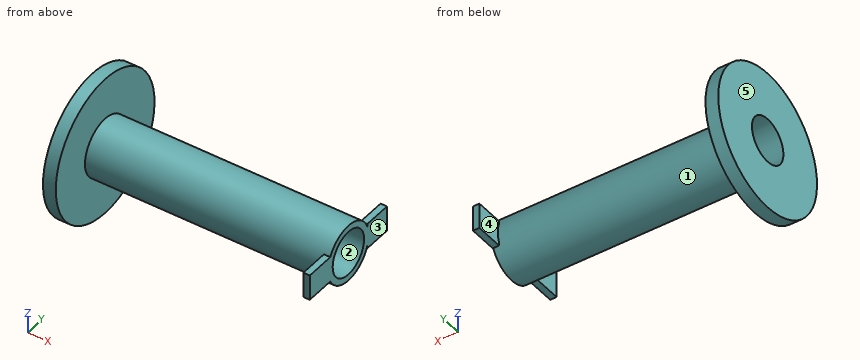
```python
from build123d import *

# Parameters (mm, degrees)
SKETCH2_R               = 55
BOSS_EXTRUDE1_DEPTH     = 10
SKETCH3_R               = 22.5
BOSS_EXTRUDE2_DEPTH     = 190
SKETCH4_R               = 17.5
CUT_EXTRUDE1_DEPTH      = 1
CUT_EXTRUDE1_DEPTH_BACK = 201
SKETCH9_W               = 20
SKETCH9_H               = 22
BOSS_EXTRUDE3_DEPTH     = 5
SKETCH10_W              = 20
SKETCH10_H              = 23
BOSS_EXTRUDE4_DEPTH     = 5


with BuildPart() as part:
    # Sketch2 → Boss-Extrude1 (new body)
    with BuildSketch(Plane(origin=(0, 0, 0), x_dir=(0, 0, -1), z_dir=(1, 0, 0))):
        Circle(SKETCH2_R)
    extrude(amount=BOSS_EXTRUDE1_DEPTH)

    # Sketch3 → Boss-Extrude2 (add)
    with BuildSketch(Plane(origin=(10, 0, 0), x_dir=(0, 0, -1), z_dir=(1, 0, 0))):
        Circle(SKETCH3_R)
    extrude(amount=BOSS_EXTRUDE2_DEPTH)

    # Sketch4 → Cut-Extrude1 (cut, two sides)
    with BuildSketch(Plane.ZY) as cut_extrude1_sk:
        Circle(SKETCH4_R)
    extrude(amount=CUT_EXTRUDE1_DEPTH, mode=Mode.SUBTRACT)
    extrude(cut_extrude1_sk.sketch, amount=-CUT_EXTRUDE1_DEPTH_BACK, mode=Mode.SUBTRACT)

    # Sketch9 → Boss-Extrude3 (add)
    with BuildSketch(Plane(origin=(200, 0, 0), x_dir=(0, 0, -1), z_dir=(1, 0, 0))):
        with Locations((0, 32)):
            Rectangle(SKETCH9_W, SKETCH9_H)
    extrude(amount=-BOSS_EXTRUDE3_DEPTH)

    # Sketch10 → Boss-Extrude4 (add)
    with BuildSketch(Plane(origin=(200, 0, 0), x_dir=(0, 0, -1), z_dir=(1, 0, 0))):
        with Locations((0, -31.5)):
            Rectangle(SKETCH10_W, SKETCH10_H)
    extrude(amount=-BOSS_EXTRUDE4_DEPTH)


solid = part.part
```
The model under review builds one solid part; all positions refer to its coordinate system, in mm. Face numbers are marked on the shaded views. A direction names the side the tool comes from. Round coordinates to 2 decimals unless told otherwise and drop trailing zeros. Loops run counter-clockwise (first coordinate to the right, second up) from the corner with the lowest first, then second, coordinate; pieces in that order, holes last. Notation, with made-up numbers: (-26, 71) - (-8, 71) arc R32 cw to (-8, 104) - close; hole circle Ø10 at (62.5, 22.25). An arc over 180 degrees is marked (long way). Use a Markdown table: item, result. Add a question column.
Q1. Add section C-C (x = 113). State the section outline as (y, z) points.
Q2. Add section D-D (y = -30). State the section outline as (x, z) points, plus the area to 3 significant figures.
Q3. Add section B-B (z = 0). State the section outline as (x, y) points, plus the area to 4 significant figures.
Q4. Add section A-A (y = 0). State the section outline as (x, z) points, plus the area to 3 significant figures.
Q5. Machinability: for the marked faces 1 and 2, which of the approach directions +Z, -Z, +X, -X, +Y, -Y give a long, thin tool a straight path to every point of the face, cutting with its end or side? Answer none if there is none.
Q6. For probe 1 along Y at (x, z) = (120.5, 0); probe 2 along X at (y, z) = (9, -42.5); probe 3 along Z at (x, y) = (18, -5), list the stretches that pass through material, from the lowest coordinate up.
Q7. Insertion check: pin 1 Ø8 at (x, z) = (88, -24) entering from -Y; pin 2 Ø4 at (x, y) = (196.5, -30) entering from +Z; pin 3 Ø1.5 at (x, z) = (198.5, 2) entering from +Y. Each pin has a flat end and moves straight along its axis. Give the tip position at first contact, or say it passes through.
Q8. The part is to be moulded in two halves that separate along X. For the marked faces 3, 4 and 5, say which applies: pulls with the +X half, pulls with the -X half, needs draft (parallel to the pull), parting line crosses it, or undercut.
Worked answers:
| question | item | result |
|---|---|---|
| 1 | outline | circle Ø45 at (0, 0); hole circle Ø35 at (0, 0) |
| 2 | outline | (0, -46.1) - (10, -46.1) - (10, 46.1) - (0, 46.1) - close; (195, -10) - (200, -10) - (200, 10) - (195, 10) - close |
| 2 | area | 1,020 mm² |
| 3 | outline | (0, -55) - (10, -55) - (10, -22.5) - (195, -22.5) - (195, -43) - (200, -43) - (200, -17.5) - (0, -17.5) - close; (0, 17.5) - (200, 17.5) - (200, 43) - (195, 43) - (195, 22.5) - (10, 22.5) - (10, 55) - (0, 55) - close |
| 3 | area | 2,855 mm² |
| 4 | outline | (0, -55) - (10, -55) - (10, -22.5) - (200, -22.5) - (200, -17.5) - (0, -17.5) - close; (0, 17.5) - (200, 17.5) - (200, 22.5) - (10, 22.5) - (10, 55) - (0, 55) - close |
| 4 | area | 2,650 mm² |
| 5 | face 1 | none |
| 5 | face 2 | +X, -X |
| 6 | probe 1 | -22.5 to -17.5, 17.5 to 22.5 |
| 6 | probe 2 | 0 to 10 |
| 6 | probe 3 | -21.94 to -16.77, 16.77 to 21.94 |
| 7 | pin 1 | y = -10.31 |
| 7 | pin 2 | z = 10 |
| 7 | pin 3 | y = 43 |
| 8 | face 3 | pulls with the +X half |
| 8 | face 4 | undercut |
| 8 | face 5 | pulls with the -X half |
